Design review of the part built by this model. Coordinates are the model's own, in mm. Give positions to 0.01 mm unless a question says otherwise; leave off trailing zeros. Order: outer loops, then holes, each group sorted by start corner. A loop starts at its lowest first (then second) coordinate and runs counter-clockwise, first axis right, second up. Notation, with made-up numbers: (-1, -28) -> (20, -28) arc R25 cw to (20, 11) -> close; hole circle Ø8 at (76.25, 10). An arc over 180 degrees is marked (long way). Use a Markdown table: item, result. Add a question column.
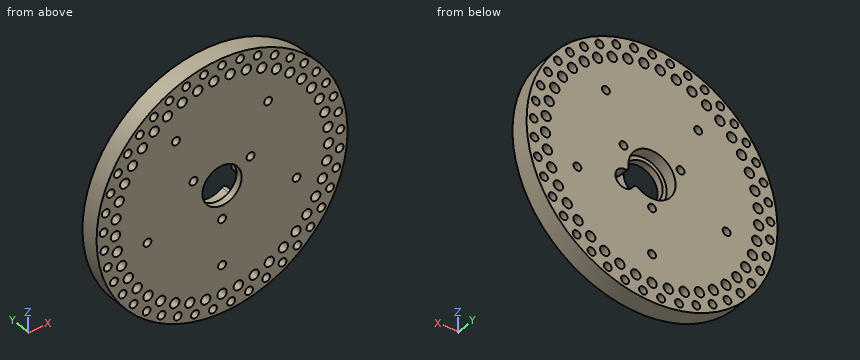
```python
from build123d import *

# Parameters (mm, degrees)
SKETCH1_R                          = 40
PODSTAWA_DEPTH                     = 6
PRZELOT_SPRZEGLA_REACH             = 58.886
SKETCH2_R                          = 7.5
PRZELOT_SPRZEGLA_DIRECTION_2_DEPTH = 57.885850613
WALKI_CYKLOIDY_D                   = 3
TAP_DRILL_FOR_M3_TAP1_D            = 2.5
PROG_START                         = 2.2
SKETCH9_R                          = 7.5
SKETCH9_R_2                        = 6.25
PROG_LOZYSKA_DEPTH                 = 2.2
TAP_DRILL_FOR_M3_TAP2_D            = 2.5
SKETCH12_R                         = 3
CUT_EXTRUDE1_DEPTH                 = 3.8
FILLET1_R                          = 1
TAP_DRILL_FOR_M3_TAP3_D            = 2.5
TAP_DRILL_FOR_M3_TAP3_DEPTH        = 6
TAP_DRILL_FOR_M3_TAP3_TIP          = 0.751075774


with BuildPart() as part:
    # Sketch1 → podstawa (new body)
    with BuildSketch(Plane(origin=(0, 0, 0), x_dir=(1, 0, 0), z_dir=(0, 1, 0))):
        with Locations(Location((0, 0, 0), (0, 0, 270))):
            Circle(SKETCH1_R)
    extrude(amount=PODSTAWA_DEPTH)

    # Sketch2 → przelot sprzegla (cut, up to next)
    with BuildSketch(Plane(origin=(0, 6, 0), x_dir=(1, 0, 0), z_dir=(0, 1, 0)), mode=Mode.PRIVATE) as przelot_sprzegla_sk1:
        with Locations(Location((0, 0, 0), (0, 0, 90))):
            Circle(SKETCH2_R)
    przelot_sprzegla_tool1 = extrude(przelot_sprzegla_sk1.sketch, amount=-PRZELOT_SPRZEGLA_REACH, mode=Mode.PRIVATE) & part.part
    add(przelot_sprzegla_tool1.solids().sort_by_distance((0, 6, 0))[0], mode=Mode.SUBTRACT)

    # Sketch2 → przelot sprzegla direction 2 (cut)
    with BuildSketch(Plane(origin=(0, 6, 0), x_dir=(1, 0, 0), z_dir=(0, 1, 0))):
        with Locations(Location((0, 0, 0), (0, 0, 90))):
            Circle(SKETCH2_R)
    extrude(amount=PRZELOT_SPRZEGLA_DIRECTION_2_DEPTH, mode=Mode.SUBTRACT)

    # walki cykloidy (through all)
    with Locations(Plane(origin=(0, 6, 0), x_dir=(1, 0, 0), z_dir=(0, 1, 0))):
        with Locations((0, 34), (5.190075663, 33.601534409), (10.258500352, 32.41547733), (15.086474487, 30.469628937), (19.560834447, 27.809598266), (23.576705027, 24.497734182), (27.039957623, 20.611663973), (29.869416531, 16.242473829), (31.998761631, 11.492573866), (33.37808288, 6.473297712), (33.975050156, 1.302292945), (33.775671052, -3.899236464), (32.784618845, -9.009371075), (31.02512296, -13.908333664), (28.538424488, -18.4812967), (25.382809535, -22.621073806), (21.632243039, -26.230632114), (17.374635101, -29.225366638), (12.709780443, -31.535083337), (7.747019303, -33.105644412), (2.602674596, -33.90023724), (-2.602674596, -33.90023724), (-7.747019303, -33.105644412), (-12.709780443, -31.535083337), (-17.374635101, -29.225366638), (-21.632243039, -26.230632114), (-25.382809535, -22.621073806), (-28.538424488, -18.4812967), (-31.02512296, -13.908333664), (-32.784618845, -9.009371075), (-33.775671052, -3.899236464), (-33.975050156, 1.302292945), (-33.37808288, 6.473297712), (-31.998761631, 11.492573866), (-29.869416531, 16.242473829), (-27.039957623, 20.611663973), (-23.576705027, 24.497734182), (-19.560834447, 27.809598266), (-15.086474487, 30.469628937), (-10.258500352, 32.41547733), (-5.190075663, 33.601534409)):
            Hole(WALKI_CYKLOIDY_D / 2)

    # Tap Drill for M3 Tap1 (through all)
    with Locations(Plane(origin=(0, 6, 0), x_dir=(1, 0, 0), z_dir=(0, 1, 0))):
        with Locations((-2.889734295, 37.639233995), (2.889734295, 37.639233995), (8.601469961, 36.757002251), (14.111594462, 35.013217529), (19.290955149, 32.448752664), (24.018152198, 29.123716538), (28.182384116, 25.116045181), (31.686044836, 20.519675013), (34.447011522, 15.442341053), (36.400569453, 10.003051708), (37.500928888, 4.329299309), (37.722298335, -1.445928197), (37.05948908, -7.187264371), (35.528036811, -12.76013716), (33.163837472, -18.033923149), (30.022305891, -22.885009264), (26.177076905, -27.199690158), (21.718279423, -30.876833369), (16.750423879, -33.830249775), (11.389952597, -35.9907138), (5.762510479, -37.307585998), (0, -37.75), (-5.762510479, -37.307585998), (-11.389952597, -35.9907138), (-16.750423879, -33.830249775), (-21.718279423, -30.876833369), (-26.177076905, -27.199690158), (-30.022305891, -22.885009264), (-33.163837472, -18.033923149), (-35.528036811, -12.76013716), (-37.05948908, -7.187264371), (-37.722298335, -1.445928197), (-37.500928888, 4.329299309), (-36.400569453, 10.003051708), (-34.447011522, 15.442341053), (-31.686044836, 20.519675013), (-28.182384116, 25.116045181), (-24.018152198, 29.123716538), (-19.290955149, 32.448752664), (-14.111594462, 35.013217529), (-8.601469961, 36.757002251)):
            Hole(TAP_DRILL_FOR_M3_TAP1_D / 2)

    # Sketch9 → prog lozyska (add)
    with BuildSketch(Plane(origin=(0, 0, 0), x_dir=(1, 0, 0), z_dir=(0, 1, 0)).offset(PROG_START)):
        with Locations(Location((0, 0, 0), (0, 0, 90))):
            Circle(SKETCH9_R)
        with Locations(Location((0, 0, 0), (0, 0, 270))):
            Circle(SKETCH9_R_2, mode=Mode.SUBTRACT)
    extrude(amount=-PROG_LOZYSKA_DEPTH)

    # Tap Drill for M3 Tap2 (through all)
    with Locations(Plane(origin=(0, 6, 0), x_dir=(1, 0, 0), z_dir=(0, 1, 0))):
        with Locations((0, 10.5), (9.09326674, -5.25), (-9.09326674, -5.25)):
            Hole(TAP_DRILL_FOR_M3_TAP2_D / 2)

    # Sketch12 → Cut-Extrude1 (cut)
    with BuildSketch(Plane(origin=(0, 6, 0), x_dir=(1, 0, 0), z_dir=(0, 1, 0))):
        with Locations((8.660254038, 5)):
            Circle(SKETCH12_R)
    extrude(amount=-CUT_EXTRUDE1_DEPTH, mode=Mode.SUBTRACT)

    # Fillet1
    fillet1_edges = [part.edges().sort_by_distance(p)[0] for p in [
        (7.090883633, 4.1, -2.443229276),
        (5.661340437, 4.1, -4.919270724),
    ]]
    fillet(fillet1_edges, radius=FILLET1_R)

    # Tap Drill for M3 Tap3
    with Locations(Plane(origin=(0, 6, 0), x_dir=(1, 0, 0), z_dir=(0, 1, 0))):
        with Locations((0, 25), (23.776412907, 7.725424859), (14.694631307, -20.225424859), (-14.694631307, -20.225424859), (-23.776412907, 7.725424859)):
            Hole(TAP_DRILL_FOR_M3_TAP3_D / 2, depth=TAP_DRILL_FOR_M3_TAP3_DEPTH)
            with Locations((0, 0, -(TAP_DRILL_FOR_M3_TAP3_DEPTH + TAP_DRILL_FOR_M3_TAP3_TIP / 2))):  # 118° drill point
                Cone(0, TAP_DRILL_FOR_M3_TAP3_D / 2, TAP_DRILL_FOR_M3_TAP3_TIP, mode=Mode.SUBTRACT)


solid = part.part
```
1) For L1, parallel to Z at x = -12.5, y = 4.75; L2, parallel to X at y = 1.75, z = 7; L3, parallel to X at y = 4.75, z = 27.5, list the stretches that pass through material, from the lowest coordinate up. Write a range as [from, to].
2) Add section A-A (x = 0). Give the boundary of the cut face in (y, z).
3) Insertion check: pin 1 (2.5 mm diameter, centred on x = 29.87, z = -16.24, fed in from -Y); pin 2 (1 mm diameter, centred on y = 5, z = -3.5, fed in from -X). Each pin has a flat end and moves straight along its axis. Give the tip position at first contact, or say it passes through.
4) Add section B-B (y = 4.75). Give the number of separate pieces and of enclosed holes in the cut face, then the cut area to 3 significant figures.
Worked answers:
| question | item | result |
|---|---|---|
| 1 | L1 | [-38, 30.05], [33.02, 35.42], [36.57, 38] |
| 1 | L2 | [-39.38, -38.3], [-35.82, 35.82], [38.3, 39.38] |
| 1 | L3 | [-29.05, -27.39], [-24.96, -22.43], [-20.83, 20.83], [22.43, 24.96], [27.39, 29.05] |
| 2 | outline | (0, -40) -> (6, -40) -> (6, -35.5) -> (0, -35.5) -> close; (0, -32.5) -> (6, -32.5) -> (6, -26.25) -> (0, -26.25) -> close; (0, -23.75) -> (6, -23.75) -> (6, -11.75) -> (0, -11.75) -> close; (0, -9.25) -> (6, -9.25) -> (6, -7.5) -> (2.2, -7.5) -> (2.2, -6.25) -> (0, -6.25) -> close; (0, 6.25) -> (2.2, 6.25) -> (2.2, 7.5) -> (6, 7.5) -> (6, 36.5) -> (0, 36.5) -> close; (0, 39) -> (6, 39) -> (6, 40) -> (0, 40) -> close |
| 3 | pin 1 | through |
| 3 | pin 2 | x = -39.89 |
| 4 | separate pieces | 1 |
| 4 | enclosed holes | 91 |
| 4 | area | 4,290 mm^2 |
